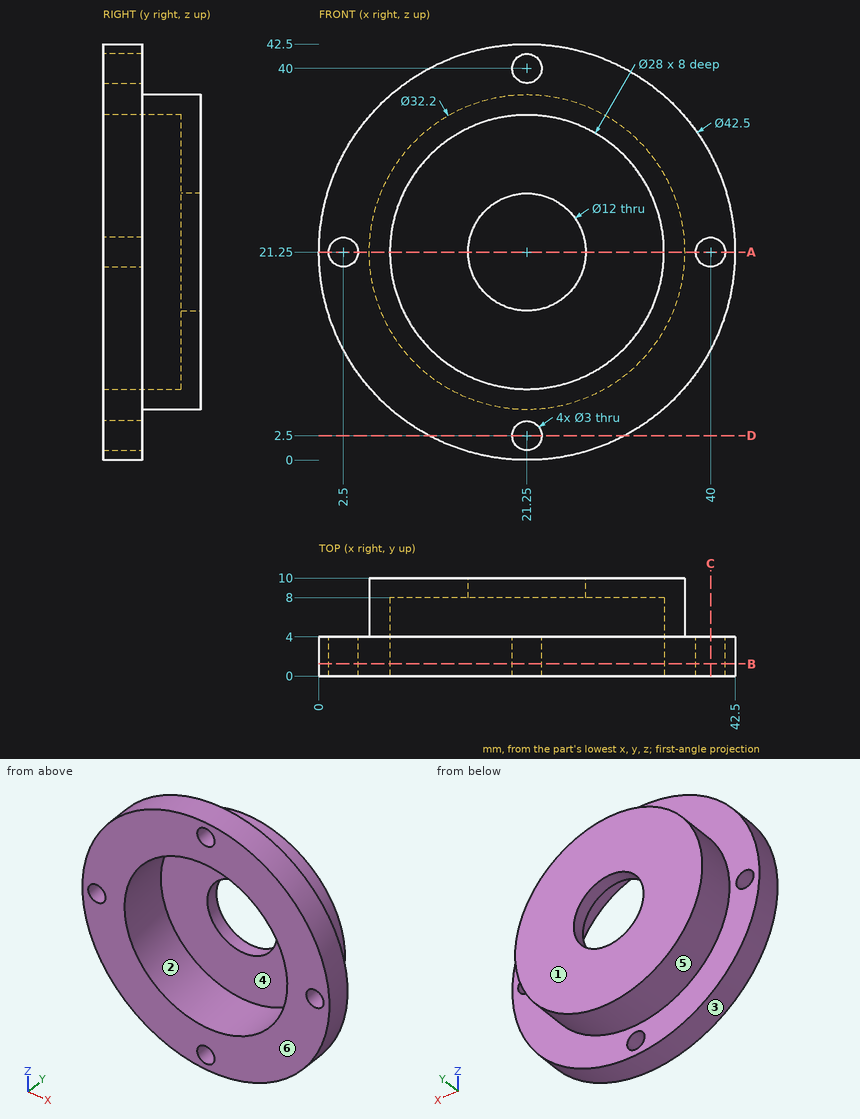
Can you work these out from the drawing? Everything is in mm from the part's minimum corner. A direction names the side the tool comes from. Round coordinates to 2 decimals unless told otherwise and drop trailing zeros. Order: outer loops, then holes, each group sorted by start corner. A loop starts at its lowest first (then second) coordinate and runs counter-clockwise, first axis right, second up. Notation, with made-up numbers: (27, -24.75) -> (61, -24.75) arc R18 cw to (61, -18.75) -> close; hole circle Ø1 at (-8, -10). An arc over 180 degrees is marked (long way). Return JSON: item names as keys, results as strings. Group by question number.
1. Which directions (+Z, -Z, +X, -X, +Y, -Y) give clear straight access to the entire face, cutting with the end or side of a thin tool? Please do the marked faces 5 and 6.
2. If we section it at B-B, the plane y = 1.25: Write out the boundary of the cut face in (x, z), then the cut area to 3 significant figures.
3. Will these pins go through, and if not, where does the flat tip stop? pin 1 (4 mm diameter, centred on y = 6.5, z = 16.5, fed in from +X); pin 2 (2 mm diameter, centred on y = 4.5, z = 22.5, fed in from +X); pin 3 (3 mm diameter, centred on x = 5, y = 7.5, fed in from -Z).
4. If we section it at D-D, the plane z = 2.5: Write out the boundary of the cut face in (x, y), then the cut area to 3 significant figures.
5. If we section it at C-C, the plane x = 40: Write out the boundary of the cut face in (y, z), then the cut area to 3 significant figures.
6. We'd pull the mould along Z, two halves only. Please class the marked faces 1, 2, 3 and 4: released by +Z, released by -Z, zero draft, split by the parting line, or undercut.
7. If we section it at A-A, the plane z = 21.25: Write out the boundary of the cut face in (x, y), then the cut area to 3 significant figures.
8. I need wall thicknesses on line 1 (X direction, y = 2.95, z = 21.25); line 2 (X direction, y = 3.25, z = 29); line 3 (Z direction, x = 12, y = 1.25). Which ranges of each line are inside material? Lowest first, please. Write a range as [from, to].
Output values:
{
 "1": {"face 5": "+Y", "face 6": "+Z, -Z, +X, -X, -Y"},
 "2": {"outline": "circle Ø42.5 at (21.25, 21.25); hole circle Ø3 at (2.5, 21.25); hole circle Ø28 at (21.25, 21.25); hole circle Ø3 at (21.25, 2.5); hole circle Ø3 at (21.25, 40); hole circle Ø3 at (40, 21.25)", "area": "775 mm²"},
 "3": {"pin 1": "x = 37.11", "pin 2": "x = 42.5", "pin 3": "z = 14.8"},
 "4": {"outline": "(11.25, 0) -> (19.75, 0) -> (19.75, 4) -> (11.25, 4) -> close; (22.75, 0) -> (31.25, 0) -> (31.25, 4) -> (22.75, 4) -> close", "area": "68.0 mm²"},
 "5": {"outline": "(0, 11.25) -> (4, 11.25) -> (4, 19.75) -> (0, 19.75) -> close; (0, 22.75) -> (4, 22.75) -> (4, 31.25) -> (0, 31.25) -> close", "area": "68.0 mm²"},
 "6": {"face 1": "zero draft", "face 2": "undercut", "face 3": "split by the parting line", "face 4": "undercut"},
 "7": {"outline": "(0, 0) -> (1, 0) -> (1, 4) -> (0, 4) -> close; (4, 0) -> (7.25, 0) -> (7.25, 8) -> (15.25, 8) -> (15.25, 10) -> (5.15, 10) -> (5.15, 4) -> (4, 4) -> close; (27.25, 8) -> (35.25, 8) -> (35.25, 0) -> (38.5, 0) -> (38.5, 4) -> (37.35, 4) -> (37.35, 10) -> (27.25, 10) -> close; (41.5, 0) -> (42.5, 0) -> (42.5, 4) -> (41.5, 4) -> close", "area": "91.2 mm²"},
 "8": {"line 1": "[0, 1], [4, 7.25], [35.25, 38.5], [41.5, 42.5]", "line 2": "[1.46, 9.59], [32.91, 41.04]", "line 3": "[2.12, 10.74], [31.76, 40.38]"}
}
